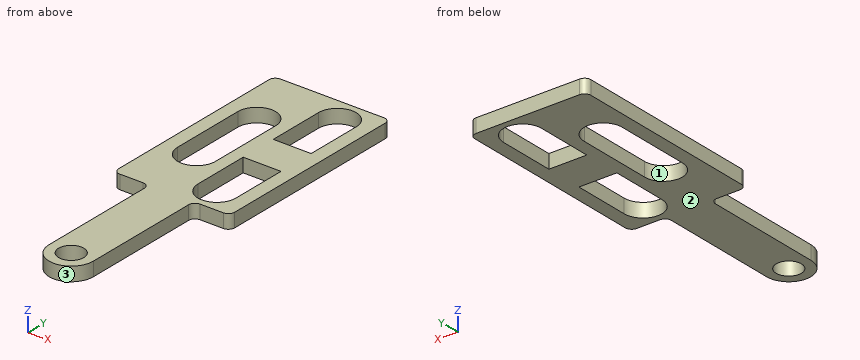
```python
from build123d import *

# Parameters (mm, degrees)
PAD_DEPTH     = 2.2
FILLET_R      = 1
SKETCH001_R   = 2
SKETCH001_R_2 = 1
POCKET_DEPTH  = 5


with BuildPart() as part:
    # Sketch → Pad (new body)
    with BuildSketch(Plane.XY):
        with BuildLine():
            Line((-9.2, 16), (9.2, 16))
            Line((9.2, 16), (9.2, -16))
            Line((9.2, -16), (4.5, -16))
            Line((4.5, -16), (4.5, -17))
            Line((4.5, -17), (3.5, -17))
            Line((3.5, -17), (3.5, -36))
            ThreePointArc((-3.5, -36), (0, -39.500021), (3.5, -36))
            Line((-3.5, -36), (-3.5, -17))
            Line((-3.5, -17), (-4.5, -17))
            Line((-4.5, -17), (-4.5, -16))
            Line((-4.5, -16), (-9.2, -16))
            Line((-9.2, -16), (-9.2, 16))
        make_face()
    extrude(amount=PAD_DEPTH)

    # Fillet
    fillet_edges = [part.edges().sort_by_distance(p)[0] for p in [
        (-9.2, 16, 1.1),
        (9.2, 16, 1.1),
        (9.2, -16, 1.1),
        (-9.2, -16, 1.1),
    ]]
    fillet(fillet_edges, radius=FILLET_R)

    # Sketch001 (on DatumPlane) → Pocket (cut)
    with BuildSketch(Plane.XY.offset(2.2)):
        with Locations((0, -36)):
            Circle(SKETCH001_R)
        with Locations((-4.5, -17)):
            Circle(SKETCH001_R_2)
        with Locations((4.5, -17)):
            Circle(SKETCH001_R_2)
        with BuildLine():
            ThreePointArc((-1, 6.00001), (-4.000005, 9.000001), (-7, 6))
            Line((-7, -6), (-7, 6))
            ThreePointArc((-7, -6), (-3.999995, -8.999997), (-1, -5.99999))
            Line((-1, -5.99999), (-1, 6.00001))
        make_face()
        with BuildLine():
            Line((1, 12), (1, 3))
            Line((1, 3), (7, 3))
            Line((7, 3), (7, 12))
            ThreePointArc((7, 12), (4, 15), (1, 12))
        make_face()
        with BuildLine():
            Line((1, -12), (1, -3))
            Line((1, -3), (7, -3))
            Line((7, -3), (7, -12))
            ThreePointArc((1, -12), (4, -15), (7, -12))
        make_face()
    extrude(amount=-POCKET_DEPTH, mode=Mode.SUBTRACT)


solid = part.part
```
Source: CAD feature listing. Evaluate the final solid. Frame: model axes, mm. Face numbers are marked on the shaded views. Round coordinates to 2 decimals unless told otherwise and drop trailing zeros. Loops run counter-clockwise (first coordinate to the right, second up) from the corner with the lowest first, then second, coordinate; pieces in that order, holes last.
1. Section query A-A on x = 4. Output: boundary loops of the cut face in (y, z), and give its area (3 significant figures).
2. Ray query, L1, parallel to X at y = 12, z = 1.8; L2, parallel to Y at x = 0, z = 0.55; L3, parallel to X at y = 0, z = 1.95. Return the intervals inside material, ascending.
3. Section query C-C on x = -4. Output: boundary loops of the cut face in (y, z), and give its area (3 significant figures).
4. Mould query, pull axis Y, two halves, no side actions, for the marked faces 1, 2 and 3. Classes: released by +Y, released by -Y, zero draft, split by the parting line, or undercut.
5. Section query D-D on y = -20. Output: boundary loops of the cut face in (x, z).
6. Section query B-B on z = 1.25. Output: boundary loops of the cut face in (x, y).
Answers below:
1. outline: (-16.13, 0) - (-15, 0) - (-15, 2.2) - (-16.13, 2.2) - close; (-3, 0) - (3, 0) - (3, 2.2) - (-3, 2.2) - close; (15, 0) - (16, 0) - (16, 2.2) - (15, 2.2) - close
1. area: 17.9 mm2
2. L1: x = -9.2 to 1, 7 to 9.2
2. L2: y = -39.5 to -38, -34 to 16
2. L3: x = -9.2 to -7, -1 to 9.2
3. outline: (-16.13, 0) - (-9, 0) - (-9, 2.2) - (-16.13, 2.2) - close; (9, 0) - (16, 0) - (16, 2.2) - (9, 2.2) - close
3. area: 31.1 mm2
4. face 1: undercut
4. face 2: zero draft
4. face 3: released by -Y
5. outline: (-3.5, 0) - (3.5, 0) - (3.5, 2.2) - (-3.5, 2.2) - close
6. outline: (-9.2, -15) arc R1 ccw to (-8.2, -16) - (-4.5, -16) arc R1 cw to (-3.5, -17) - (-3.5, -36) arc R3.5 ccw to (3.5, -36) - (3.5, -17) arc R1 cw to (4.5, -16) - (8.2, -16) arc R1 ccw to (9.2, -15) - (9.2, 15) arc R1 ccw to (8.2, 16) - (-8.2, 16) arc R1 ccw to (-9.2, 15) - close; hole (-7, -6) arc R3 ccw to (-1, -6) - (-1, 6) arc R3 ccw to (-7, 6) - close; hole circle Ø4 at (0, -36); hole (1, -12) arc R3 ccw to (7, -12) - (7, -3) - (1, -3) - close; hole (1, 3) - (7, 3) - (7, 12) arc R3 ccw to (1, 12) - close
